Geometry: final body of the model. Coordinates: model frame, mm. A direction names the side the tool comes from. Round coordinates to 2 decimals unless told otherwise and drop trailing zeros. Write each loop counter-clockwise with the first axis right and the second up, starting at its lowest first coordinate (ties: lowest second). Pieces come first, ordered by that corner, then holes. Notation, with made-up numbers: M 36.5,76 L 48.5,76 A19 ccw 48.5,105 Z; hole C 5,57 d9. An arc over 180 degrees is marked long. Use one line per item in the form item = value. Start each with the question number.
Item 1: Section query A-A (x = 32). Return loops of the section in (y, z), and give its area (3 significant figures).
Item 2: Pull-direction query (Y, two-part tool) for faces 1 (the flat face through (-13.955, 24.171, 1.479)), 2 (the cylindrical face through (5.22, -16.61, 1.48)), 3 (the flat face through (0.9, -11.3, 0)), 4 (the cylindrical face through (37.47, -20.14, 1.48)); classes: pulls with the +Y half, pulls with the -Y half, needs draft (parallel to the pull), parting line crosses it, or undercut.
Item 3: Ray query, probe 1 along X at (y, z) = (-8, 1.95); probe 2 along Y at (x, z) = (-26, 0.85); probe 3 along X at (y, z) = (34.5, 1.35). Return the intervals inside material, ascending.
Item 4: Section query C-C (y = 34). Return loops of the section in (x, z).
Item 5: Section query D-D (z = 1.7). Return loops of the section in (x, y).
Item 6: Section query B-B (y = -18.5). Return loops of the section in (x, z), and give its area (3 significant figures).
Item 7: Reachability of faces 5 (the flat face through (11.041, 24.125, 1.479)), 6 (the flat face through (15.37, -21.62, 1.48)), 7 (the flat face through (0.9, -11.3, 3)), 8 (the cylindrical face through (-36.176, -22.382, 1.479)), 9 (the flat face through (28, 0, 1)) from +Z, -Z, +X, -X, +Y, -Y: full face, straight path, thin tool, end or side. Return the list, or none.
Item 8: Pin query (flat end, axial travel): pin 1 Ø1 at (y, z) = (14, 2) entering from -X; pin 2 Ø12 at (x, y) = (0, 32.65) entering from +Z. Return the tip coordinate at first contact, or that it passes through.
from build123d import *

# Parameters (mm, degrees)
F0_R     = 9.95
F1_DEPTH = 3


with BuildPart() as f1:
    # F0 (on Top) → F1 (new body)
    with BuildSketch(Plane.XY):
        with BuildLine():
            Line((7.244864, 15.831038), (14.943939, 32.654589))
            ThreePointArc((14.943939, 32.654589), (9.53394, 41.597928), (0, 45.882246))
            ThreePointArc((0, 45.882246), (-11.930072, 43.001993), (-19.059785, 33.012515))
            Line((-19.059785, 33.012515), (-8.705025, 15.077545))
            ThreePointArc((-8.705025, 15.077545), (-12.310764, 12.310764), (-15.077545, 8.705025))
            ThreePointArc((-15.077545, 8.705025), (-17.010717, 3.70747), (-17.332513, -1.641283))
            Line((-17.332513, -1.641283), (-35.751673, -3.385464))
            ThreePointArc((-35.751673, -3.385464), (-38.884293, -24.666016), (-19.059785, -33.012515))
            Line((-19.059785, -33.012515), (-8.705025, -15.077545))
            ThreePointArc((-8.705025, -15.077545), (-4.506052, -16.816817), (0, -17.41005))
            ThreePointArc((0, -17.41005), (5.294595, -16.585448), (10.087649, -14.189756))
            Line((10.087649, -14.189756), (20.807735, -29.269125))
            ThreePointArc((20.807735, -29.269125), (40.803543, -21.341778), (38.119569, 0))
            Line((38.119569, 0), (17.41005, 0))
            ThreePointArc((17.41005, 0), (16.816817, 4.506052), (15.077545, 8.705025))
            ThreePointArc((15.077545, 8.705025), (11.716122, 12.877978), (7.244864, 15.831038))
        make_face()
        with Locations((-28.279704, -16.327295)):
            Circle(F0_R, mode=Mode.SUBTRACT)
        with BuildLine():
            ThreePointArc((-9.526279, 5.5), (0, 11), (9.526279, 5.5))
            ThreePointArc((9.526279, 5.5), (9.526279, -5.5), (0, -11))
            ThreePointArc((0, -11), (-9.526279, -5.5), (-9.526279, 5.5))
        make_face(mode=Mode.SUBTRACT)
        with Locations((28.279704, -16.327295)):
            Circle(F0_R, mode=Mode.SUBTRACT)
        with Locations((0, 32.654589)):
            Circle(F0_R, mode=Mode.SUBTRACT)
    extrude(amount=F1_DEPTH)


solid = f1.part
Working result:
q1.outline = M -28.79,0 L -25.56,0 L -25.56,3 L -28.79,3 Z; M -7.1,0 L 0,0 L 0,3 L -7.1,3 Z
q1.area = 31.0 mm²
q2.face_1 = undercut
q2.face_2 = pulls with the -Y half
q2.face_3 = needs draft
q2.face_4 = undercut
q3.probe_1 = -39.19 to -33.73, -22.83 to -7.55, 7.55 to 22.83, 33.73 to 42.69
q3.probe_2 = -33.44 to -26.01, -6.64 to -2.46
q3.probe_3 = -18.59 to -9.78, 9.78 to 14.38
q4.outline = M -18.76,0 L -9.86,0 L -9.86,3 L -18.76,3 Z; M 9.86,0 L 14.55,0 L 14.55,3 L 9.86,3 Z
q5.outline = M -35.75,-3.39 A17.56 ccw -19.06,-33.01 L -8.71,-15.08 A17.41 ccw 0,-17.41 A17.41 ccw 10.09,-14.19 L 20.81,-29.27 A17.56 ccw 38.12,0 L 17.41,0 A17.41 ccw 15.08,8.71 A17.41 ccw 7.24,15.83 L 14.94,32.65 A17.56 ccw 0,45.88 A17.56 ccw -19.06,33.01 L -8.71,15.08 A17.41 ccw -15.08,8.71 A17.41 ccw -17.33,-1.64 Z; hole C -28.28,-16.33 d19.9; hole C 0,0 d22; hole C 0,32.65 d19.9; hole C 28.28,-16.33 d19.9
q6.outline = M -40.97,0 L -37.99,0 L -37.99,3 L -40.97,3 Z; M -18.57,0 L -10.68,0 L -10.68,3 L -18.57,3 Z; M 13.15,0 L 18.57,0 L 18.57,3 L 13.15,3 Z; M 37.99,0 L 42.16,0 L 42.16,3 L 37.99,3 Z
q6.area = 61.4 mm²
q7.face_5 = +Z, -Z, +X
q7.face_6 = +Z, -Z, -Y
q7.face_7 = +Z, +X, -X, +Y, -Y
q7.face_8 = +Z, -Z
q7.face_9 = +Z, -Z, +X, +Y
q8.pin_1 = -10.99
q8.pin_2 = through
